For this review, take the finished solid that the model builds, in its own axes (mm). Give positions to 0.01 mm unless a question says otherwise; leave off trailing zeros. Order: outer loops, then holes, each group sorted by start corner. A loop starts at its lowest first (then second) coordinate and runs counter-clockwise, first axis right, second up. Notation, with made-up numbers: (5, 16.25) - (19, 16.25) arc R16 cw to (19, 21.25) - close; hole circle Ø8 at (61, -25.5). An arc over 180 degrees is marked (long way). Use a Markdown table: item, result. Add a question column.
1) We need section D-D on x = -51. Write out the cut boundary in (y, z), then the cut area to 3 significant figures.
2) We need section A-A on z = 0. Write out the cut boundary in (x, y), then the cut area to 3 significant figures.
3) Wall thickness on L1, parallel to Y at x = 119, z = 0; L2, parallel to Y at x = 136, z = 0; L3, parallel to Z at x = 94.5, y = 314: over which ranges is each line inside the solid? List them lowest first.
4) Clearance check with flat-ended pins moving along their axes: P1, Ø2, axis at x = -66, y = 421.5, coming from the -Z side; P2, Ø5, axis at x = -33.5, z = -189, coming from the +Y side; P3, Ø1.5, axis at x = 96, z = 509, coming from the -Y side. State where each tip first meets the part, or that it passes through.
5) We need section C-C on x = 16. Write out the cut boundary in (y, z).
```python
from build123d import *

# Parameters (mm, degrees)
FILLET2_R = 21


with BuildPart() as part:
    # Sketch1 → Revolve1 (revolve)
    with BuildSketch(Plane.XY, mode=Mode.PRIVATE) as revolve1_sk:
        with BuildLine():
            Line((155, 530), (89.4427191, 530))
            ThreePointArc((89.4427191, 530), (0, 570), (-89.4427191, 530))
            Line((-89.4427191, 530), (-155, 530))
            Line((-155, 530), (-155, 650))
            Line((-155, 650), (155, 650))
            Line((155, 650), (155, 530))
        make_face()
    revolve(revolve1_sk.sketch.rotate(Axis((-124.426605505, 0, 0), (1, 0, 0)), 90), axis=Axis((-124.426605505, 0, 0), (1, 0, 0)))

    # Fillet2
    fillet2_edges = [part.edges().sort_by_distance(p)[0] for p in [
        (155, 0, -650),
        (-155, 0, -650),
    ]]
    fillet(fillet2_edges, radius=FILLET2_R)


solid = part.part
```
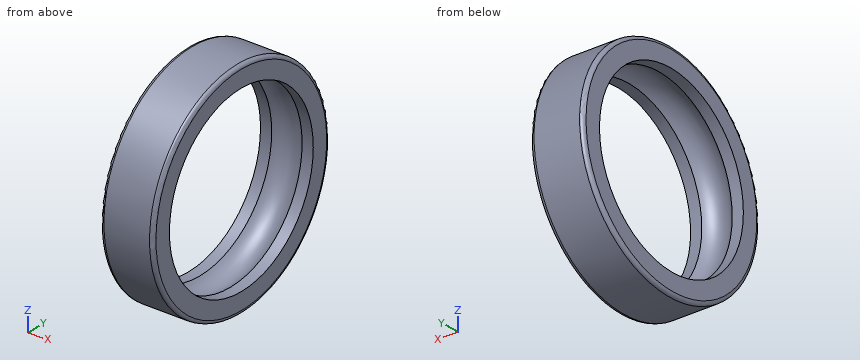
Checked values:
| question | item | result |
|---|---|---|
| 1 | outline | circle Ø1300 at (0, 0); hole circle Ø1117.25 at (0, 0) |
| 1 | area | 347,000 mm² |
| 2 | outline | (-155, -629) arc R21 ccw to (-134, -650) - (134, -650) arc R21 ccw to (155, -629) - (155, -530) - (89.44, -530) arc R120 cw to (-89.44, -530) - (-155, -530) - close; (-155, 530) - (-89.44, 530) arc R120 cw to (89.44, 530) - (155, 530) - (155, 629) arc R21 ccw to (134, 650) - (-134, 650) arc R21 ccw to (-155, 629) - close |
| 2 | area | 64,100 mm² |
| 3 | L1 | -650 to -530, 530 to 650 |
| 3 | L2 | -649.9 to -530, 530 to 649.9 |
| 3 | L3 | -569.13 to -426.97, 426.97 to 569.13 |
| 4 | P1 | z = -495.66 |
| 4 | P2 | y = 622.67 |
| 4 | P3 | y = -405.19 |
| 5 | outline | circle Ø1300 at (0, 0); hole circle Ø1137.86 at (0, 0) |
